Print and shaded views of the part. All mm, measured from the part's lowest x, y and z. A direction names the side the tool comes from. Coordinates: 2 decimals unless noted, no trailing zeros. Loops run counter-clockwise (first coordinate to the right, second up) from the corner with the lowest first, then second, coordinate; pieces in that order, holes last. Notation, with made-up numbers: (-31.5, 10) -> (-21.5, 10) arc R7 ccw to (-21.5, 18) -> close; hole circle Ø2 at (31.25, -21). An arc over 180 degrees is marked (long way). One line per question, with ' | ' between items. Start each with the question number.
1) 3-axis set-ups, long thin cutter, end or side, ignore diameter. For the marked faces 1, 2 and 3: which of +Z, -Z, +X, -X, +Y, -Y reach the whole face in a straight line?
2) Cut at A-A (y = 156.5). List the corners of the cut face in (x, z), plus the area to 3 significant figures.
3) Drop a flat-ended pin along its axis: pin 1 (4 mm diameter, centred on x = 626.5, y = 77, fed in from -Z). Give the stop position or say it passes through.
4) Cut at B-B (z = 288). List the corners of the cut face in (x, y).
5) Cut at C-C (x = 599). List the corners of the cut face in (y, z), plus the area to 3 significant figures.
6) Probe L1, parallel to X at y = 231, z = 101.5; L2, parallel to Y at x = 497, z = 355. List the from-to ranges inside material, lowest first. Write a range as from..to.
7) Cut at D-D (z = 637.5). List the corners of the cut face in (x, y).
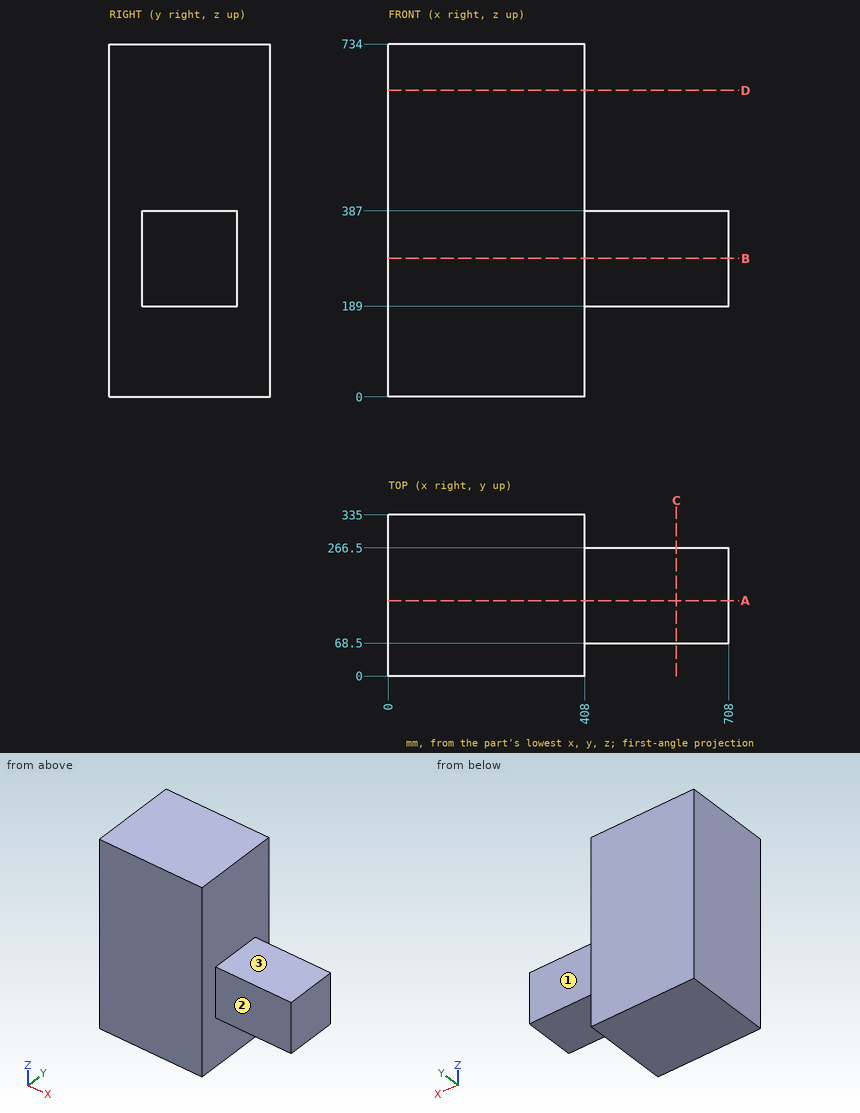
Reported:
1) face 1: +Z, -Z, +X, +Y | face 2: +Z, -Z, +X, -Y | face 3: +Z, +X, +Y, -Y
2) outline: (0, 0) -> (408, 0) -> (408, 189) -> (708, 189) -> (708, 387) -> (408, 387) -> (408, 734) -> (0, 734) -> close | area: 359,000 mm²
3) pin 1: stops at z = 189
4) outline: (0, 0) -> (408, 0) -> (408, 68.5) -> (708, 68.5) -> (708, 266.5) -> (408, 266.5) -> (408, 335) -> (0, 335) -> close
5) outline: (68.5, 189) -> (266.5, 189) -> (266.5, 387) -> (68.5, 387) -> close | area: 39,200 mm²
6) L1: x = 0..408 | L2: y = 68.5..266.5
7) outline: (0, 0) -> (408, 0) -> (408, 335) -> (0, 335) -> close
